The model under review builds one solid part; all positions refer to its coordinate system, in mm. Face numbers are marked on the shaded views. A direction names the side the tool comes from. Coordinates: 2 decimals unless noted, no trailing zeros. Write each loop counter-clockwise with the first axis right and the second up, starting at its lowest first coordinate (ties: lowest second). Pieces come first, ordered by that corner, then holes. Notation, with made-up numbers: (33.5, 86.25) - (72.5, 86.25) arc R25 cw to (72.5, 119.25) - close; hole circle Ø10 at (72.25, 44.5). An arc over 180 degrees is marked (long way). Put each result on its own line as item: value. Start each with the question number.
Item 1: Consider section A-A on x = -2. Give the boundary of the cut face in (y, z) (3 decimals).
Item 2: Mouldability with a two-part tool opening along Y and no side actions: class the marked faces 4, 5, 6 and 7 as pulls with the +Y half, pulls with the -Y half, needs draft (parallel to the pull), parting line crosses it, or undercut.
Item 3: For pin 1 (8.5 mm diameter, centred on y = -0.5, z = 1.5, fed in from -X); pin 2 (1 mm diameter, centred on x = -1.5, y = -0.5, fed in from -Z); pin 3 (12 mm diameter, centred on x = 5, y = 10, fed in from +Z), all flat-tipped, find the tip position at first contact; note any pin that passes through.
Item 4: Machinability: for the marked faces 1, 2 and 3, which of the approach directions +Z, -Z, +X, -X, +Y, -Y give a long, thin tool a straight path to every point of the face, cutting with its end or side? Answer none if there is none.
Item 5: To check wall thickness, follow L1, parallel to X at y = -6.25, z = 12.75; L2, parallel to Y at x = -0.75, z = 0; L3, parallel to Y at x = 4.25, z = -1.5. State the ranges of each line that lie inside material, in increasing order. Write a range as [from, to].
Item 6: Consider section B-B on x = 7.25. Give the boundary of the cut face in (y, z), then the cut area to 3 significant figures.
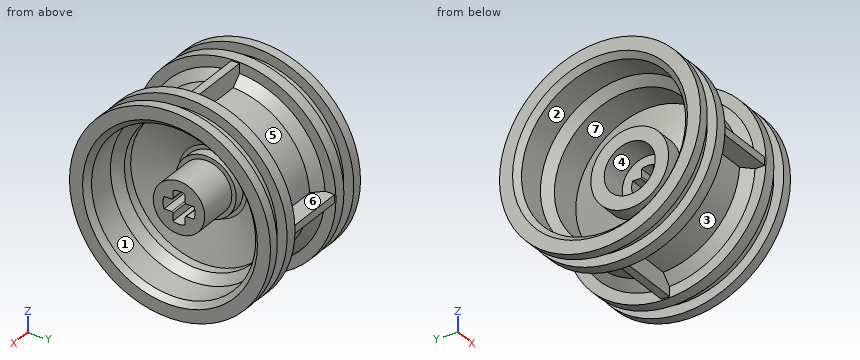
```python
from build123d import *

# Parameters (mm, degrees)
CUT_EXTRUDE2_REACH = 29.821
RIB1_REACH         = 25.452
SKETCH7_WALL_W     = 58.004157598
SKETCH7_WALL_H     = 1.2
CIRPATTERN1_COUNT  = 4
CHAMFER1_SIZE      = 0.8


with BuildPart() as part:
    # Sketch1 → Revolve1 (revolve)
    with BuildSketch(Plane.XY, mode=Mode.PRIVATE) as revolve1_sk:
        Polygon((10, 12.25), (10, 15), (8.5, 15), (8.5, 13.5), (6.31, 13.5), (6.31, 15), (4.55, 15), (4.55, 13.375), (3.175, 12), (-3.175, 12), (-4.55, 13.375), (-4.55, 15), (-6.31, 15), (-6.31, 13.5), (-8.5, 13.5), (-8.5, 15), (-10, 15), (-10, 12.25), (-5, 12.25), (-3.75, 11), (3.75, 11), (5, 12.25), align=None)
    revolve(revolve1_sk.sketch.rotate(Axis((0, 0, 0), (1, 0, 0)), 90), axis=Axis((0, 0, 0), (1, 0, 0)))

    # Sketch2 → Revolve3 (revolve)
    with BuildSketch(Plane.XY, mode=Mode.PRIVATE) as revolve3_sk:
        Polygon((1, 11), (2.37, 11), (0.5, 5.1), (0.5, 4.5), (2, 4.5), (2, 3.85), (8, 3.85), (8, 0), (0.6, 0), (0.6, 3.804964539), (-3.4, 3.804964539), (-3.4, 5.8), (-0.648135593, 5.8), align=None)
    revolve(revolve3_sk.sketch.rotate(Axis((0, 0, 0), (1, 0, 0)), 90), axis=Axis((0, 0, 0), (1, 0, 0)))

    # Sketch5 → Cut-Extrude2 (cut, up to next)
    with BuildSketch(Plane(origin=(8, 0, 0), x_dir=(0, 0, -1), z_dir=(1, 0, 0)), mode=Mode.PRIVATE) as cut_extrude2_sk1:
        with BuildLine():
            Line((0.9, 1.1), (0.9, 2.224859546))
            ThreePointArc((0.9, 2.224859546), (0, 2.4), (-0.9, 2.224859546))
            Line((-0.9, 2.224859546), (-0.9, 1.1))
            ThreePointArc((-0.9, 1.1), (-0.958578644, 0.958578644), (-1.1, 0.9))
            Line((-1.1, 0.9), (-2.224859546, 0.9))
            ThreePointArc((-2.224859546, 0.9), (-2.4, 0), (-2.224859546, -0.9))
            Line((-2.224859546, -0.9), (-1.1, -0.9))
            ThreePointArc((-1.1, -0.9), (-0.958578644, -0.958578644), (-0.9, -1.1))
            Line((-0.9, -1.1), (-0.9, -2.224859546))
            ThreePointArc((-0.9, -2.224859546), (0, -2.4), (0.9, -2.224859546))
            Line((0.9, -2.224859546), (0.9, -1.1))
            ThreePointArc((0.9, -1.1), (0.958578644, -0.958578644), (1.1, -0.9))
            Line((1.1, -0.9), (2.224859546, -0.9))
            ThreePointArc((2.224859546, -0.9), (2.4, 0), (2.224859546, 0.9))
            Line((2.224859546, 0.9), (1.1, 0.9))
            ThreePointArc((1.1, 0.9), (0.958578644, 0.958578644), (0.9, 1.1))
        make_face()
    cut_extrude2_tool1 = extrude(cut_extrude2_sk1.sketch, amount=-CUT_EXTRUDE2_REACH, mode=Mode.PRIVATE) & part.part
    add(cut_extrude2_tool1.solids().sort_by_distance((8, 0, 0))[0], mode=Mode.SUBTRACT)

    # Sketch7 wall → Rib1 (add, up to next)
    with BuildSketch(Plane(origin=(0, 14.8, 0), x_dir=(-1, 0, 0), z_dir=(0, -1, 0)), mode=Mode.PRIVATE) as rib1_sk1:
        Rectangle(SKETCH7_WALL_W, SKETCH7_WALL_H)
    rib1_tool1 = extrude(rib1_sk1.sketch, amount=RIB1_REACH, mode=Mode.PRIVATE) - part.part
    rib1 = rib1_tool1.solids().sort_by_distance((0, 14.8, 0))[0]
    add(rib1)

    # CirPattern1: Rib1 ×4 about axis
    cirpattern1_axis = Axis((0, 0, 0), (1, 0, 0))
    for i in range(1, CIRPATTERN1_COUNT):
        add(rib1.rotate(cirpattern1_axis, i * 360 / CIRPATTERN1_COUNT))

    # Chamfer1
    chamfer1_edges = [part.edges().sort_by_distance(p)[0] for p in [
        (10, 0, -12.25),
        (-10, 0, -12.25),
    ]]
    chamfer(chamfer1_edges, length=CHAMFER1_SIZE)


solid = part.part
```
Report:
1. outline: (-14.8, -0.6) - (-11.985, -0.6) arc R12 ccw to (-0.6, -11.985) - (-0.6, -14.8) - (0.6, -14.8) - (0.6, -11.985) arc R12 ccw to (11.985, -0.6) - (14.8, -0.6) - (14.8, 0.6) - (11.985, 0.6) arc R12 ccw to (0.6, 11.985) - (0.6, 14.8) - (-0.6, 14.8) - (-0.6, 11.985) arc R12 ccw to (-11.985, 0.6) - (-14.8, 0.6) - close; circle Ø11.6 at (0, 0); hole circle Ø22 at (0, 0); hole circle Ø7.61 at (0, 0)
2. face 4: undercut
2. face 5: pulls with the +Y half
2. face 6: needs draft
2. face 7: undercut
3. pin 1: x = -3.4
3. pin 2: z = -14.8
3. pin 3: z = 14.46
4. face 1: +X
4. face 2: -X
4. face 3: -Z, -Y
5. L1: [-10, -8.5], [-6.31, -4.55], [4.55, 6.31], [8.5, 10]
5. L2: [-14.8, -11], [-5.8, -3.8], [3.8, 5.8], [11, 14.8]
5. L3: [-12.99, -11.4], [-3.55, -0.9], [0.9, 3.55], [11.4, 12.99]
6. outline: circle Ø27 at (0, 0); circle Ø7.7 at (0, 0); hole circle Ø24.5 at (0, 0); hole (-2.22, -0.9) - (-1.1, -0.9) arc R0.2 cw to (-0.9, -1.1) - (-0.9, -2.22) arc R2.4 ccw to (0.9, -2.22) - (0.9, -1.1) arc R0.2 cw to (1.1, -0.9) - (2.22, -0.9) arc R2.4 ccw to (2.22, 0.9) - (1.1, 0.9) arc R0.2 cw to (0.9, 1.1) - (0.9, 2.22) arc R2.4 ccw to (-0.9, 2.22) - (-0.9, 1.1) arc R0.2 cw to (-1.1, 0.9) - (-2.22, 0.9) arc R2.4 ccw to start
6. area: 134 mm²
